Model file for the job. Use its own axes, mm. A direction names the side the tool comes from. Give positions to 0.01 mm unless a question says otherwise; leave off trailing zeros. Loops run counter-clockwise (first coordinate to the right, second up) from the corner with the lowest first, then second, coordinate; pieces in that order, holes last. Notation, with made-up numbers: M 34,66 L 55,66 A33 cw 55,97 Z; hole C 32.25,-20 d10. An arc over 180 degrees is marked long. Answer in a Markdown table with one row per item.
```python
from build123d import *

# Parameters (mm, degrees)
BOSS_EXTRUDE2_DEPTH = 2
FILLET1_R           = 1.2


with BuildPart() as part:
    # Sketch1 → Boss-Extrude2 (new body)
    with BuildSketch(Plane(origin=(0, 0, 0), x_dir=(1, 0, 0), z_dir=(0, 1, 0))):
        with BuildLine():
            Line((4.974937186, 7.5), (10, 7.5))
            ThreePointArc((10, 7.5), (-12.5, 0), (10, -7.5))
            Line((10, -7.5), (4.974937186, -7.5))
            ThreePointArc((4.974937186, -7.5), (-9, 0), (4.974937186, 7.5))
        make_face()
    extrude(amount=BOSS_EXTRUDE2_DEPTH)

    # Fillet1
    fillet1_edges = [part.edges().sort_by_distance(p)[0] for p in [
        (10, 1, 7.5),
        (10, 1, -7.5),
    ]]
    fillet(fillet1_edges, radius=FILLET1_R)


solid = part.part
```
Q1. Saw through at D-D (z = 0). Give the cut face in (x, y), and give its area (3 significant figures).
Reported:
| item | result |
|---|---|
| outline | M -12.5,0 L -9,0 L -9,2 L -12.5,2 Z |
| area | 7.00 mm² |
Q2. 3-axis set-ups, long thin cutter, end or side, ignore diameter. For faces 4 (the face through (-9.1, 0, -1)), 5 (the face through (6, 1, 7.5)): which of +Z, -Z, +X, -X, +Y, -Y reach the whole face in a straight line?
Reported:
| item | result |
|---|---|
| face 4 | +Z, -Z, +X, -X, -Y |
| face 5 | +X, +Y, -Y |
Q3. Drop flat-ended pins along their axis: pin 1 (11 mm diameter, centred on x = 0, z = 0, fed in from -Y); pin 2 (1 mm diameter, centred on x = 6.5, y = 1.5, fed in from -Z). Give the stop position or say it passes through.
Reported:
| item | result |
|---|---|
| pin 1 | through |
| pin 2 | z = -10.97 |
Q4. Saw through at B-B (y = 1.35). Give the cut face in (x, z), and give its area (3 significant figures).
Reported:
| item | result |
|---|---|
| outline | M 4.97,-7.5 A9 cw long 4.97,7.5 L 7.21,7.5 A1.2 ccw 7.98,9.62 A12.5 ccw long 7.98,-9.62 A1.2 ccw 7.21,-7.5 Z |
| area | 174 mm² |
Q5. Saw through at C-C (x = 4). Give the cut face in (y, z), and give its area (3 significant figures).
Reported:
| item | result |
|---|---|
| outline | M 0,-11.84 L 2,-11.84 L 2,-8.06 L 0,-8.06 Z; M 0,8.06 L 2,8.06 L 2,11.84 L 0,11.84 Z |
| area | 15.1 mm² |
Q6. Probe probe 1 along Z at (x, y) = (0, 1); probe 2 along Z at (x, y) = (-6.5, 0.7); probe 3 along X at (y, z) = (0.7, 0). List the from-to ranges inside material, lowest first.
Reported:
| item | result |
|---|---|
| probe 1 | -12.5 to -9, 9 to 12.5 |
| probe 2 | -10.68 to -6.22, 6.22 to 10.68 |
| probe 3 | -12.5 to -9 |
Q7. Saw through at A-A (x = 0). Give the cut face in (y, z), and give its area (3 significant figures).
Reported:
| item | result |
|---|---|
| outline | M 0,-12.5 L 2,-12.5 L 2,-9 L 0,-9 Z; M 0,9 L 2,9 L 2,12.5 L 0,12.5 Z |
| area | 14.0 mm² |
Q8. Mould opens along Z. For faces 1 (the face through (-9, 1, 0)), 2 (the face through (-9.1, 2, -1)), 3 (the face through (-12.494, 0.986, -0.396)) say: released by +Z, released by -Z, zero draft, split by the parting line, or undercut.
Reported:
| item | result |
|---|---|
| face 1 | undercut |
| face 2 | zero draft |
| face 3 | split by the parting line |
